Verification items for the finished model (mm, model axes). Face numbers are marked on the shaded views. A direction names the side the tool comes from. Coordinates: 2 decimals unless noted, no trailing zeros. Loops run counter-clockwise (first coordinate to the right, second up) from the corner with the lowest first, then second, coordinate; pieces in that order, holes last. Notation, with made-up numbers: (85, 49) -> (103, 49) arc R9 cw to (103, 58) -> close; hole circle Ø8 at (34.25, 80). An arc over 180 degrees is marked (long way). Answer as a JSON object with one key per item and string values. Group by question number.
Q1. Set-up check for the marked faces 1 and 2: record each of +Z, -Z, +X, -X, +Y, -Y from which the full face is reachable in a straight line by a thin tool's end or side.
Q2. Cross-section at B-B on x = -6. Record the boundary of the cut face in (y, z).
Q3. Gauge pin test, flat ends, axial feed: pin 1 Ø15 at (x, z) = (-11.5, 5.5) entering from +Y; pin 2 Ø2.5 at (x, y) = (-1, 7) entering from +Z; pin 3 Ø4 at (x, y) = (-4.5, 7.5) entering from -Z. Record the tip position at first contact, or that the pin passes through.
Q4. Scan lines: L1, parallel to Y at x = -1.5, z = 13.5; L2, parallel to Z at x = 26, y = 6; L3, parallel to Y at x = 9, z = -15. Record each from-to range of solid material in increasing order.
Q5. Cross-section at C-C on y = 7.25. Record the boundary of the cut face in (x, z).
Q6. Cross-section at D-D on x = 6. Record the boundary of the cut face in (y, z), and give its area (3 significant figures).
Q7. Cross-section at A-A on z = -5.5. Record the boundary of the cut face in (x, y).
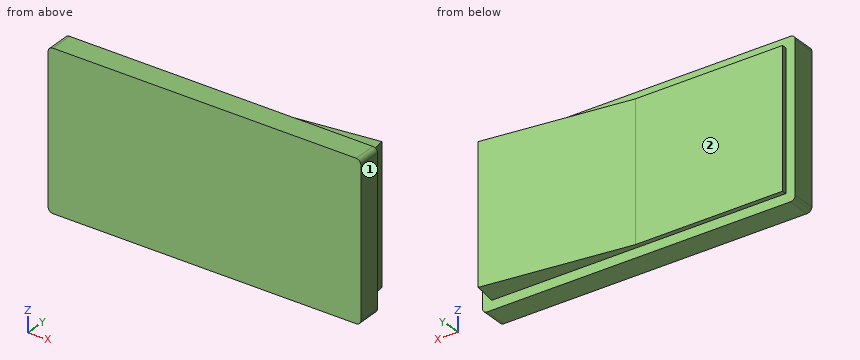
```python
from build123d import *

# Parameters (mm, degrees)
SKETCH1_W               = 67
SKETCH1_H               = 33.5
BOSS_EXTRUDE1_DEPTH     = 5
FILLET1_R               = 1
SKETCH2_W               = 63
SKETCH2_H               = 29.5
BOSS_EXTRUDE2_DEPTH     = 5
CUT_EXTRUDE1_DEPTH      = 3
CUT_EXTRUDE1_DEPTH_BACK = 32.5


with BuildPart() as part:
    # Sketch1 → Boss-Extrude1 (new body)
    with BuildSketch(Plane(origin=(0, 0, 0), x_dir=(1, 0, 0), z_dir=(0, 1, 0))):
        Rectangle(SKETCH1_W, SKETCH1_H)
    extrude(amount=BOSS_EXTRUDE1_DEPTH)

    # Fillet1
    fillet1_edges = [part.edges().sort_by_distance(p)[0] for p in [
        (33.5, 2.5, 16.75),
        (-33.5, 2.5, 16.75),
        (-33.5, 2.5, -16.75),
        (33.5, 2.5, -16.75),
    ]]
    fillet(fillet1_edges, radius=FILLET1_R)

    # Sketch2 → Boss-Extrude2 (add)
    with BuildSketch(Plane(origin=(0, 5, 0), x_dir=(1, 0, 0), z_dir=(0, 1, 0))):
        Rectangle(SKETCH2_W, SKETCH2_H)
    extrude(amount=BOSS_EXTRUDE2_DEPTH)

    # Sketch3 → Cut-Extrude1 (cut, two sides)
    with BuildSketch(Plane.XY.offset(14.75)) as cut_extrude1_sk:
        Polygon((-31.5, 6), (0, 6), (30.851738311, 10), (-31.5, 10), align=None)
        Polygon((31.5, 10), (30.851738311, 10), (31.5, 5), align=None)
    extrude(amount=CUT_EXTRUDE1_DEPTH, mode=Mode.SUBTRACT)
    extrude(cut_extrude1_sk.sketch, amount=-CUT_EXTRUDE1_DEPTH_BACK, mode=Mode.SUBTRACT)


solid = part.part
```
Computed values:
{
 "1": {"face 1": "+Z, -Z, +X, +Y, -Y", "face 2": "+Z, -Z, -X, +Y"},
 "2": {"outline": "(0, -16.75) -> (5, -16.75) -> (5, -14.75) -> (6, -14.75) -> (6, 14.75) -> (5, 14.75) -> (5, 16.75) -> (0, 16.75) -> close"},
 "3": {"pin 1": "stops at y = 6", "pin 2": "stops at z = 14.75", "pin 3": "stops at z = -14.75"},
 "4": {"L1": "y = 0 to 6", "L2": "z = -14.75 to 14.75", "L3": "y = 0 to 5"},
 "5": {"outline": "(9.64, -14.75) -> (31.21, -14.75) -> (31.21, 14.75) -> (9.64, 14.75) -> close"},
 "6": {"outline": "(0, -16.75) -> (5, -16.75) -> (5, -14.75) -> (6.78, -14.75) -> (6.78, 14.75) -> (5, 14.75) -> (5, 16.75) -> (0, 16.75) -> close", "area": "220 mm²"},
 "7": {"outline": "(-33.5, 0) -> (33.5, 0) -> (33.5, 5) -> (31.5, 5) -> (30.85, 10) -> (0, 6) -> (-31.5, 6) -> (-31.5, 5) -> (-33.5, 5) -> close"}
}
